Check sheet for the modelled part. Datum: model origin and axes. Units: mm. Round coordinates to 2 decimals unless told otherwise and drop trailing zeros. Write each loop counter-clockwise with the first axis right and the second up, starting at its lowest first coordinate (ties: lowest second). Pieces come first, ordered by that corner, then holes.
Item 1: Material ranges on line 1 (X direction, y = 5, z = -9); line 2 (X direction, y = 5.5, z = -77.5); line 3 (X direction, y = 5, z = -15.25), recorded low to high.
Item 2: Go/stop test with flat-tipped pins: pin 1 Ø2.5 at (x, y) = (-220, 5) entering from -Z; pin 2 Ø3.5 at (x, y) = (-150, 5) entering from +Z; pin 3 Ø3.5 at (y, z) = (5, -220) entering from +X. Record where each tip stops, or that it passes through.
Item 3: Cross-section at B-B on x = -102.5. Enter the section's corners in (y, z).
Item 4: Cross-section at C-C on z = -280.5. Enter the section's corners in (x, y), plus the area to 3 significant figures.
Item 5: Cross-section at A-A on z = -232.5. Enter the section's corners in (x, y), plus the area to 3 significant figures.
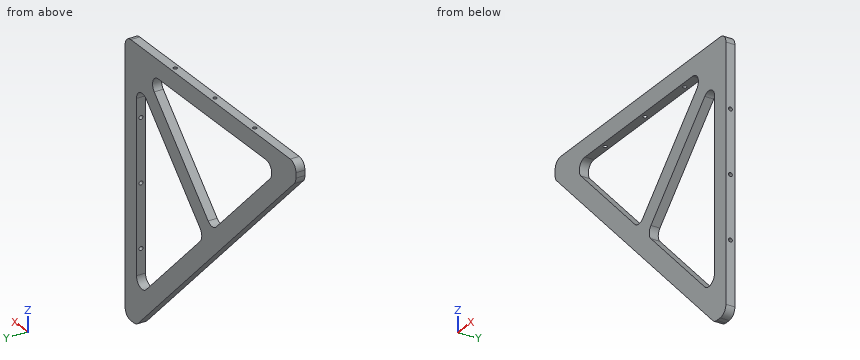
Autodesk Inventor part; units mm, degrees
ref_plane "YZ Plane" through (0, 0, 0) normal (1, 0, 0) x (0, 1, 0)
ref_plane "XZ Plane" through (0, 0, 0) normal (0, 1, 0) x (-1, 0, 0)
ref_plane "XY Plane" through (0, 0, 0) normal (0, 0, 1) x (1, 0, 0)
sketch "Sketch1" plane through (0, 0, 0) normal (0, 1, 0) x (-1, 0, 0)
  line L0 (0, 0) -> (20, 0)
  line L1 (20, 0) -> (20, -300)
  line L2 (20, -300) -> (0, -300)
  line L3 (0, -300) -> (0, 0)
  line L4 (0, 0) -> (300, 0)
  line L5 (300, 0) -> (300, -20)
  line L6 (300, -20) -> (0, -20)
  line L7 (0, -20) -> (0, 0)
  line L8 (300, -20) -> (20, -300)
  line L9 (285.8579, -5.8579) -> (5.8579, -285.8579)
  line L10 (-7.0711, -7.0711) -> (152.9289, -167.0711)
  line L11 (7.0711, 7.0711) -> (167.0711, -152.9289)
  point P0 (138.7868, -152.9289)
  point P1 (20, -271.7157)
  point P2 (20, -34.1421)
  point P3 (152.9289, -138.7868)
  point P4 (34.1421, -20)
  point P5 (271.7157, -20)
  dimension "d32" = 20
  dimension "d33" = 300
  dimension "d34" = 300
  dimension "d35" = 20
  dimension "d36" = 20
extrude "Extrusion1" add sketch "Sketch1" along normal blind 10 contours L0 L11 L1 L6 L10 L3 | L0 L1 L11 | L10 L6 L3 | L4 L5 L6 L11 L1 | L11 L6 L1 | L6 L10 L1 L2 L3 | L6 L1 L10 | L6 L11 L9 L10 L1 | L8 L11 L9 L6 | L11 L8 L10 L9 | L1 L9 L10 L8
fillet "Fillet1" radius 10 11 edges at (-300, 5, 0) (-300, 5, -20) (-271.7157, 5, -20) (-152.9289, 5, -138.7868) (-138.7868, 5, -152.9289) (-34.1421, 5, -20) (-20, 5, -34.1421) (0, 5, 0) (-20, 5, -300) (0, 5, -300) (-20, 5, -271.7157)
sketch "Sketch3" plane through (-290, 0, 0) normal (0, 0, 1) x (1, 0, 0)
  line L0 (0, 0) -> (0, 10)
  line L1 (0, 5) -> (70, 5)
  line L2 (70, 5) -> (140, 5)
  line L3 (140, 5) -> (210, 5)
  line L4 (210, 5) -> (280, 5)
  point P0 (290, 0)
  dimension "d39" = 70
  dimension "d40" = 70
  dimension "d41" = 70
  dimension "d42" = 70
hole "Hole2" at (-220, 5, 0) at (-150, 5, 0) at (-80, 5, 0) direction (0, 0, -1) diameter 4.3 depth 20
sketch "Sketch4" plane through (0, 0, -10) normal (1, 0, 0) x (0, 0, -1)
  line L0 (280, 10) -> (280, 0)
  line L1 (280, 5) -> (210, 5)
  line L2 (210, 5) -> (140, 5)
  line L3 (140, 5) -> (70, 5)
  line L4 (70, 5) -> (0, 5)
  point P0 (-10, 0)
  dimension "d50" = 70
  dimension "d51" = 70
  dimension "d52" = 70
  dimension "d53" = 70
hole "Hole3" at (0, 5, -220) at (0, 5, -150) at (0, 5, -80) direction (-1, 0, 0) diameter 4.3 depth 20
properties part number "Aufhängung_Gerüst"
Response values:
1. line 1: x = -299.95 to -222.15, -217.85 to -152.15, -147.85 to -82.15, -77.85 to -0.05
1. line 2: x = -242.5 to -214.22, -91.64 to -63.36, -20 to 0
1. line 3: x = -300 to -222.15, -217.85 to -152.15, -147.85 to -82.15, -77.85 to 0
2. pin 1: stops at z = -101.25
2. pin 2: stops at z = -133.48
2. pin 3: stops at x = -69.97
3. outline: (0, -217.5) - (10, -217.5) - (10, -189.22) - (0, -189.22) - close; (0, -116.64) - (10, -116.64) - (10, -88.36) - (0, -88.36) - close; (0, -20) - (10, -20) - (10, 0) - (0, 0) - close
4. outline: (-39.5, 0) - (0, 0) - (0, 10) - (-39.5, 10) - close
4. area: 395 mm2
5. outline: (-87.5, 0) - (-59.22, 0) - (-59.22, 10) - (-87.5, 10) - close; (-20, 0) - (0, 0) - (0, 10) - (-20, 10) - close
5. area: 483 mm2
